from build123d import *

# Parameters (mm, degrees)
EXTRUDE_1_DEPTH          = 40
CUT_EXTRUDE_1_DEPTH      = 19
CUT_EXTRUDE_START        = -19
CUT_EXTRUDE_2_DEPTH      = 19
CUT_EXTRUDE_3_DEPTH      = 622.369455316
CUT_EXTRUDE_4_DEPTH      = 622.369455316
CUT_EXTRUDE_4_DEPTH_BACK = 622.369455316
SKETCH_5_R               = 10.007014795


with BuildPart() as part:
    # 草图1 → 凸台-拉伸1 (new body)
    with BuildSketch(Plane.XY):
        with BuildLine():
            Line((245, 0), (245, 290.473750966))
            ThreePointArc((245, 290.473750966), (0, 380), (-245, 290.473750966))
            Line((-245, 290.473750966), (-245, 0))
            Line((-245, 0), (-225, 0))
            Line((-225, 0), (-225, 258.975090072))
            ThreePointArc((-225, 258.975090072), (0, 180), (225, 258.975090072))
            Line((225, 258.975090072), (225, 0))
            Line((225, 0), (245, 0))
        make_face()
    extrude(amount=EXTRUDE_1_DEPTH)

    # 草图2 → 切除-拉伸1 (cut)
    with BuildSketch(Plane(origin=(0, 0, 0), x_dir=(-1, 0, 0), z_dir=(0, 0, -1))):
        with BuildLine():
            Line((225, 258.975090072), (225, 281.024909928))
            ThreePointArc((225, 281.024909928), (0, 360), (-225, 281.024909928))
            Line((-225, 281.024909928), (-225, 258.975090072))
            ThreePointArc((-225, 258.975090072), (0, 180), (225, 258.975090072))
        make_face()
    extrude(amount=-CUT_EXTRUDE_1_DEPTH, mode=Mode.SUBTRACT)

    # 草图3 → 切除-拉伸2 (cut)
    with BuildSketch(Plane.XY.offset(40).offset(CUT_EXTRUDE_START)):
        with BuildLine():
            Line((225, 258.975090072), (225, 281.024909928))
            ThreePointArc((225, 281.024909928), (0, 360), (-225, 281.024909928))
            Line((-225, 281.024909928), (-225, 258.975090072))
            ThreePointArc((-225, 258.975090072), (0, 180), (225, 258.975090072))
        make_face()
    extrude(amount=CUT_EXTRUDE_2_DEPTH, mode=Mode.SUBTRACT)

    # 草图4 → 切除-拉伸3 (cut, through all)
    with BuildSketch(Plane(origin=(245, 0, 0), x_dir=(0, 0, -1), z_dir=(1, 0, 0))):
        with BuildLine():
            ThreePointArc((-20, 0), (-34.142135624, 5.857864376), (-40, 20))
            Line((-40, 20), (-40, 0))
            Line((-40, 0), (-20, 0))
        make_face()
        with BuildLine():
            ThreePointArc((0, 20), (-5.857864376, 5.857864376), (-20, 0))
            Line((-20, 0), (0, 0))
            Line((0, 0), (0, 20))
        make_face()
    extrude(amount=-CUT_EXTRUDE_3_DEPTH, mode=Mode.SUBTRACT)

    # 草图5 → 切除-拉伸4 (cut, two sides: drawn at the far end of the back side and taken through both)
    with BuildSketch(Plane.ZY.offset(245).offset(-CUT_EXTRUDE_4_DEPTH_BACK)):
        with Locations(Location((20, 20, 0), (0, 0, 270))):
            Circle(SKETCH_5_R)
    extrude(amount=CUT_EXTRUDE_4_DEPTH + CUT_EXTRUDE_4_DEPTH_BACK, mode=Mode.SUBTRACT)


solid = part.part
Verification items for the finished model (mm, model axes). A direction names the side the tool comes from. Round coordinates to 2 decimals unless told otherwise and drop trailing zeros. Order: outer loops, then holes, each group sorted by start corner. A loop starts at its lowest first (then second) coordinate and runs counter-clockwise, first axis right, second up. Notation, with made-up numbers: (-29, 33) -> (-5, 33) arc R18 cw to (-5, 66) -> close; hole circle Ø6 at (44, 89). An arc over 180 degrees is marked (long way). Put each result on its own line as item: value.
1) Section check D-D (x = 27). Record the cut outline in (y, z), then the cut area to 3 significant figures.
Final values:
outline: (181.01, 19) -> (358.99, 19) -> (358.99, 0) -> (379.04, 0) -> (379.04, 40) -> (358.99, 40) -> (358.99, 21) -> (181.01, 21) -> close
area: 1,160 mm^2
2) Material ranges on line 1 (X direction, y = 259.5, z = 36.5); line 2 (X direction, y = 250, z = 20.5); line 3 (Z direction, x = 238.75, y = 20), recorded low to high.
Final values:
line 1: x = -245 to -225, 225 to 245
line 2: x = -245 to -225, -213.31 to 213.31, 225 to 245
line 3: z = 0 to 9.99, 30.01 to 40
3) Section check C-C (y = 264.5). Record the cut outline in (x, z), then the cut area to 3 significant figures.
Final values:
outline: (-245, 0) -> (-225, 0) -> (-225, 19) -> (225, 19) -> (225, 0) -> (245, 0) -> (245, 40) -> (225, 40) -> (225, 21) -> (-225, 21) -> (-225, 40) -> (-245, 40) -> close
area: 2,500 mm^2
4) Depth check by flat-ended pin: pin 1 (6 mm diameter, centred on x = -76, z = 30, fed in from +Y); pin 2 (6 mm diameter, centred on x = 177.5, y = 233, fed in from -Z); pin 3 (4 mm diameter, centred on x = -5, y = 327.5, fed in from +Z). Enter the tip coordinate at first touch or a pass-through.
Final values:
pin 1: stops at y = 372.92
pin 2: stops at z = 19
pin 3: stops at z = 21
5) Set-up check for faces 1 (the flat face through (-3, 271, 21)), 2 (the cylindrical face through (-3.403, 359.984, 9.367)), 3 (the cylindrical face through (3.73, 379.98, 19.72)): record each of +Z, -Z, +X, -X, +Y, -Y from which the full face is reachable in a straight line by a thin tool's end or side.
Final values:
face 1: +Z, -Y
face 2: -Z, -Y
face 3: +Z, -Z, +Y
6) Section check B-B (y = 208.5). Record the cut outline in (x, z).
Final values:
outline: (-245, 0) -> (-225, 0) -> (-225, 40) -> (-245, 40) -> close; (-140.38, 19) -> (140.38, 19) -> (140.38, 21) -> (-140.38, 21) -> close; (225, 0) -> (245, 0) -> (245, 40) -> (225, 40) -> close
7) Section check A-A (y = 126). Record the cut outline in (x, z).
Final values:
outline: (-245, 0) -> (-225, 0) -> (-225, 40) -> (-245, 40) -> close; (225, 0) -> (245, 0) -> (245, 40) -> (225, 40) -> close
8) Mould release check, pull along Z, two halves, no side actions. Record for faces 4 (the flat face through (-1, 361, 40)), 5 (the flat face through (-245, 147, 20)), 6 (the cylindrical face through (235.14, 10.455, 23.006)): +Z half, -Z half, draft (parallel to the pull), parting line (faces both ways), or undercut.
Final values:
face 4: +Z half
face 5: draft
face 6: undercut
